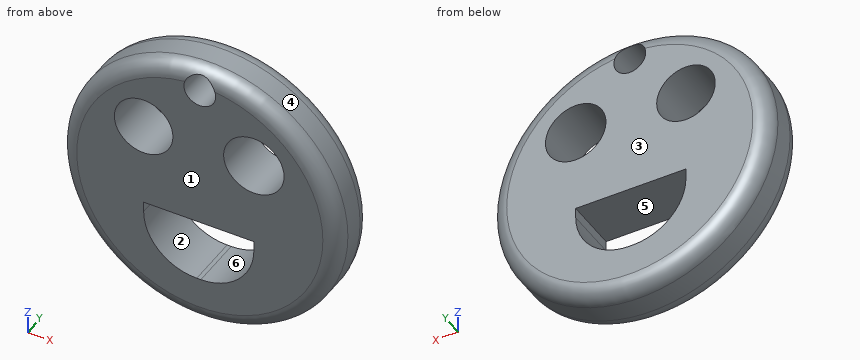
```python
from build123d import *

# Parameters (mm, degrees)
F0_R     = 26.177757608
F0_R_2   = 5.5155489558
F0_R_3   = 2.9897173108
F0_R_4   = 5.6935154322
F1_DEPTH = 10


# Not quite as in the source:
# - a fillet or chamfer that OpenCascade refuses, or shapes differently, is made with other operations: its cross-section is extruded or revolved along the edge and cut away or added


with BuildPart() as f1:
    # F0 (on Front) → F1 (new body)
    with BuildSketch(Plane.XZ):
        Circle(F0_R)
        with BuildLine():
            Line((-10.5765974149, -7.333868891), (-10.5765974149, -5.3862300701))
            Line((-10.5765974149, -5.3862300701), (10.1848710328, -5.3862300701))
            Line((10.1848710328, -5.3862300701), (10.1848710328, -7.333868891))
            ThreePointArc((10.1848710328, -7.333868891), (7.2559388447, -14.4049367029), (0.1848710328, -17.333868891))
            Line((0.1848710328, -17.333868891), (-0.5765974149, -17.333868891))
            ThreePointArc((-0.5765974149, -17.333868891), (-7.6476652268, -14.4049367029), (-10.5765974149, -7.333868891))
        make_face(mode=Mode.SUBTRACT)
        with Locations((-10.5765974149, 10.4786651209)):
            Circle(F0_R_2, mode=Mode.SUBTRACT)
        with Locations((0, 22.0345780253)):
            Circle(F0_R_3, mode=Mode.SUBTRACT)
        with Locations((10.1848710328, 10.4786651209)):
            Circle(F0_R_4, mode=Mode.SUBTRACT)
    extrude(amount=F1_DEPTH)

    # F2: fillet of radius 3 on 2 edges, made by hand

    # F2_s1 → F2_t2 (revolve, cut)
    with BuildSketch(Plane.XY):
        with BuildLine():
            ThreePointArc((26.177757608, -7), (25.2990779516, -9.1213203436), (23.177757608, -10))
            Line((23.177757608, -10), (26.177757608, -10))
            Line((26.177757608, -10), (26.177757608, -7))
        make_face()
    revolve(axis=Axis((0, -10, 0), (0, -1, 0)), mode=Mode.SUBTRACT)

    # F2_s3 → F2_t4 (revolve, cut)
    with BuildSketch(Plane.XY):
        with BuildLine():
            ThreePointArc((26.177757608, -3), (25.2990779516, -0.8786796564), (23.177757608, 0))
            Line((23.177757608, 0), (26.177757608, 0))
            Line((26.177757608, 0), (26.177757608, -3))
        make_face()
    revolve(axis=Axis((0, 0, 0), (0, -1, 0)), mode=Mode.SUBTRACT)


solid = f1.part
```
Input: part model. Units: mm. Frame: model coordinates. Face numbers are marked on the shaded views. A direction names the side the tool comes from. Coordinates: 2 decimals unless noted, no trailing zeros. Write each loop counter-clockwise with the first axis right and the second up, starting at its lowest first coordinate (ties: lowest second). Pieces come first, ordered by that corner, then holes.
1) Section A-A on y = -1. Output: boundary loops of the cut face in (x, z), and give its area (3 significant figures).
2) Set-up query: the marked faces 1 and 2. Return all of +Z, -Z, +X, -X, +Y, -Y with unobstructed straight access to the full face (end or side cutting, diameter ignored); none if empty.
3) Material intervals for line 1 along Z through (x, y) = (0, -3.5); line 2 along X through (y, z) = (-7.5, 7.5); line 3 along X through (y, z) = (-3.5, 7), sorted ascending.
4) Pin query (flat end, axial travel): pin 1 Ø6 at (x, y) = (-2.5, -9) entering from -Z; pin 2 Ø2 at (y, z) = (-7.5, -6.5) entering from -X; pin 3 Ø2 at (x, y) = (16.5, -4) entering from +Z. Return the tip coordinate at first contact, or that it passes through.
5) Mould query, pull axis Z, two halves, no side actions, for the marked faces 3, 4, 5 and 6. Classes: pulls with the +Z half, pulls with the -Z half, needs draft (parallel to the pull), parting line crosses it, or undercut.
6) Section B-B on x = -2. State how many separate pieces and enclosed holes the cut face has, and give its area (3 significant figures).
7) Section C-C on y = -4.75. Output: boundary loops of the cut face in (x, z).
Check result:
1. outline: circle Ø50.83 at (0, 0); hole circle Ø11.03 at (-10.58, 10.48); hole (-10.58, -7.33) arc R10 ccw to (-0.58, -17.33) - (0.18, -17.33) arc R10 ccw to (10.18, -7.33) - (10.18, -5.39) - (-10.58, -5.39) - close; hole circle Ø5.98 at (0, 22.03); hole circle Ø11.39 at (10.18, 10.48)
1. area: 1,600 mm2
2. face 1: +Z, -Z, +X, -X, -Y
2. face 2: +Y, -Y
3. line 1: z = -26.18 to -17.33, -5.39 to 19.04, 25.02 to 26.18
3. line 2: x = -25.04 to -15.22, -5.93 to 5.33, 15.04 to 25.04
3. line 3: x = -25.22 to -14.86, -6.3 to 5.68, 14.69 to 25.22
4. pin 1: stops at z = -26.18
4. pin 2: stops at x = -25.58
4. pin 3: stops at z = 21.1
5. face 3: needs draft
5. face 4: parting line crosses it
5. face 5: undercut
5. face 6: undercut
6. separate pieces: 3
6. enclosed holes: 0
6. area: 352 mm2
7. outline: circle Ø52.36 at (0, 0); hole circle Ø11.03 at (-10.58, 10.48); hole (-10.58, -7.33) arc R10 ccw to (-0.58, -17.33) - (0.18, -17.33) arc R10 ccw to (10.18, -7.33) - (10.18, -5.39) - (-10.58, -5.39) - close; hole circle Ø5.98 at (0, 22.03); hole circle Ø11.39 at (10.18, 10.48)
